The model under review builds one solid part; all positions refer to its coordinate system, in mm. Face numbers are marked on the shaded views. A direction names the side the tool comes from. Coordinates: 2 decimals unless noted, no trailing zeros. Write each loop counter-clockwise with the first axis right and the second up, starting at its lowest first coordinate (ties: lowest second). Pieces come first, ordered by that corner, then holes. Notation, with made-up numbers: (48, 68) - (59, 68) arc R18 cw to (59, 82) - close; hole circle Ø9 at (-33, -29). An arc over 180 degrees is marked (long way). Return JSON: item names as keys, results as strings. Group by question number.
(1) Tool access review of the marked faces 1 and 2: name each direction out of +Z, -Z, +X, -X, +Y, -Y from which nothing blocks a thin tool from reaching the whole face with its end or side.
(2) We need section A-A on z = -74. State the section outline as (x, y) points, then the cut area to 3 significant figures.
(3) For pin 1 Ø8 at (x, y) = (21, -31.5) entering from -Z; pin 2 Ø10 at (x, z) = (103.5, -74) entering from +Y; pin 3 Ø4 at (x, z) = (33, -74.5) entering from +Y, all flat-tipped, find the tip position at first contact; note any pin that passes through.
(4) Draft analysis for pull direction X (two halves, no side actions). For the marked faces 3, 4, 5 and 6, state which applies: released by +X, released by -X, zero draft, split by the parting line, or undercut.
(5) We need section C-C on y = 21.5. State the section outline as (x, z) points.
(6) To check wall thickness, follow L1, parallel to X at y = 4.5, z = -3; L2, parallel to Z at x = 97.5, y = 23.5; L3, parallel to Y at x = 77, z = 18. State the ranges of each line that lie inside material, in increasing order. Write a range as from..to.
(7) We need section D-D on z = -24.5. State the section outline as (x, y) points.
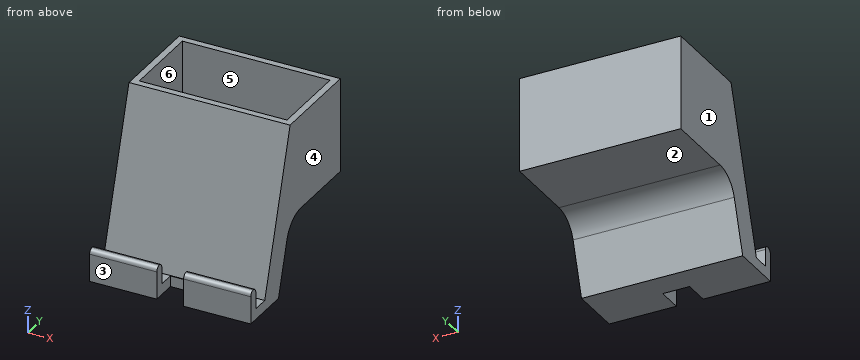
```python
from build123d import *

# Parameters (mm, degrees)
F0_W     = 70
F0_H     = 70
F1_DEPTH = 120
F2_W     = 110
F2_H     = 60
F3_DEPTH = 65
F4_W     = 20
F4_H     = 24.0523201227
F5_DEPTH = 19
F6_R     = 20.5517549394
F7_R     = 3.49999


# Not quite as in the source:
# - a fillet or chamfer is up to 0.001 mm smaller than in the source, because OpenCascade refuses the exact size


with BuildPart() as f1:
    # F0 (on Right) → F1 (new body)
    with BuildSketch(Plane.YZ):
        with Locations((0.0956673622, -2.5781301591)):
            Rectangle(F0_W, F0_H)
        Polygon((-34.9043326378, -37.5781301591), (-34.9043326378, 32.4218698409), (-70.1899622679, -82.3540924191), (-82.6712690592, -82.3540924191), (-82.6712690592, -66.3017722964), (-89.6712690592, -66.3017722964), (-89.6712690592, -82.3540924191), (-89.6712690592, -90.3540924191), (-70.1899622679, -90.3540924191), (-51.1292722594, -90.3540924191), align=None)
    extrude(amount=F1_DEPTH)

    # F2 (on face) → F3 (cut)
    with BuildSketch(Plane.XY.offset(32.4218698409)):
        with Locations((60, 0.0956673622)):
            Rectangle(F2_W, F2_H)
    extrude(amount=-F3_DEPTH, mode=Mode.SUBTRACT)

    # F4 (on face) → F5 (cut)
    with BuildSketch(Plane.XZ.offset(89.6712690592)):
        with Locations((60, -78.3279323578)):
            Rectangle(F4_W, F4_H)
    extrude(amount=-F5_DEPTH, mode=Mode.SUBTRACT)

    # F6
    f6_edges = [f1.edges().sort_by_distance(p)[0] for p in [
        (60, -34.904333, -37.57813),
    ]]
    fillet(f6_edges, radius=F6_R)

    # F7 (radius 3.5 in the source; OpenCascade refuses exactly that, so slightly less here)
    f7_edges = [f1.edges().sort_by_distance(p)[0] for p in [
        (95, -82.671269, -66.301772),
        (25, -82.671269, -66.301772),
        (25, -89.671269, -66.301772),
        (95, -89.671269, -66.301772),
    ]]
    fillet(f7_edges, radius=F7_R)


solid = f1.part
```
Ans:
{
 "1": {"face 1": "+Z, -Z, -X, +Y, -Y", "face 2": "-Z, +X, -X, +Y"},
 "2": {"outline": "(0, -89.67) - (50, -89.67) - (50, -82.67) - (0, -82.67) - close; (0, -67.62) - (120, -67.62) - (120, -46.1) - (0, -46.1) - close; (70, -89.67) - (120, -89.67) - (120, -82.67) - (70, -82.67) - close", "area": "3,280 mm²"},
 "3": {"pin 1": "z = -44.96", "pin 2": "y = -44.56", "pin 3": "y = -45.64"},
 "4": {"face 3": "zero draft", "face 4": "released by +X", "face 5": "undercut", "face 6": "undercut"},
 "5": {"outline": "(0, -37.58) - (120, -37.58) - (120, 32.42) - (115, 32.42) - (115, -32.58) - (5, -32.58) - (5, 32.42) - (0, 32.42) - close"},
 "6": {"L1": "0..5, 115..120", "L2": "-37.58..-32.58", "L3": "-39.34..-29.9, 30.1..35.1"},
 "7": {"outline": "(0, -52.4) - (120, -52.4) - (120, 35.1) - (0, 35.1) - close; hole (5, -29.9) - (115, -29.9) - (115, 30.1) - (5, 30.1) - close"}
}
